Could you check a few things on this model? Use its own coordinates, in mm. Face numbers are marked on the shaded views. A direction names the side the tool comes from. Coordinates: 2 decimals unless noted, no trailing zeros. Loops run counter-clockwise (first coordinate to the right, second up) from the corner with the lowest first, then second, coordinate; pieces in that order, holes last. Notation, with made-up numbers: (45, 6.5) -> (53, 6.5) arc R19 cw to (53, 38.5) -> close; hole circle Ø11 at (44, -37.5). An arc over 180 degrees is marked (long way). One line per question, with ' | ' between items.
from build123d import *

# Parameters (mm, degrees)
CUT_EXTRUDE1_REACH                  = 16.116
CUT_EXTRUDE1_END_RADIUS             = 2.5
CUT_EXTRUDE1_DIRECTION_2_REACH      = 16.116
CUT_EXTRUDE1_DIRECTION_2_END_RADIUS = 2.5


with BuildPart() as part:
    # Sketch2 → Revolve1 (revolve)
    with BuildSketch(Plane.XY):
        with BuildLine():
            Line((3.217141588, 1.1), (4.774934555, 1.1))
            ThreePointArc((4.774934555, 1.1), (4.9, 0), (4.774934555, -1.1))
            Line((4.774934555, -1.1), (3.217141588, -1.1))
            ThreePointArc((3.217141588, -1.1), (3.4, 0), (3.217141588, 1.1))
        make_face()
    revolve(axis=Axis((0, 4.071851736, 0), (0, -1, 0)))

    # Sketch3 → Revolve2 (revolve)
    with BuildSketch(Plane(origin=(0, 0, 0), x_dir=(1, 0, 0), z_dir=(0, 1, 0))):
        with BuildLine():
            Line((-13, 1.5), (-5.974934555, 1.5))
            Line((-5.974934555, 1.5), (-5.974934555, 0))
            Line((-5.974934555, 0), (-4.774934555, 0))
            ThreePointArc((-4.774934555, 0), (-4.594847185, 1.298991664), (-4.068169121, 2.5))
            Line((-4.068169121, 2.5), (-13, 2.5))
            Line((-13, 2.5), (-13, 1.5))
        make_face()
    revolve(axis=Axis((-1.070003769, 0, 0), (-1, 0, 0)))

    # Cut-Extrude1: up to this cylinder (the profile starts inside it)
    cut_extrude1_end = Plane(origin=(-4.461396, 0, 0), z_dir=(1, 0, 0)) * Cylinder(CUT_EXTRUDE1_END_RADIUS, 38.232024, mode=Mode.PRIVATE)
    # Sketch5 → Cut-Extrude1 (cut, up to the surface)
    with BuildSketch(Plane.XY, mode=Mode.PRIVATE) as cut_extrude1_sk1:
        with BuildLine():
            Line((-5.802324208, 2.5), (-3.740894424, 2.5))
            Line((-3.740894424, 2.5), (-3.740894424, 1.1))
            Line((-3.740894424, 1.1), (-4.646504062, 1.1))
            add(Edge.make_bspline(
                [(-4.646504062, 1.1), (-4.808494897, 1.1), (-5.037328654, 1.452538147), (-5.179468889, 2.019128522), (-5.472528246, 2.5), (-5.802324208, 2.5)],
                knots=[0, 0, 0, 0, 0.209972055, 0.594973977, 1, 1, 1, 1], degree=3))
        make_face()
    cut_extrude1_tool1 = extrude(cut_extrude1_sk1.sketch, amount=-CUT_EXTRUDE1_REACH, mode=Mode.PRIVATE) & cut_extrude1_end
    add(cut_extrude1_tool1.solids().sort_by_distance((-4.461384, 1.858771, 0))[0], mode=Mode.SUBTRACT)
    # Sketch5 → Cut-Extrude1 (cut, up to the surface)
    with BuildSketch(Plane.XY, mode=Mode.PRIVATE) as cut_extrude1_sk2:
        with BuildLine():
            Line((-3.740894424, -1.1), (-4.646504062, -1.1))
            add(Edge.make_bspline(
                [(-4.646504062, -1.1), (-4.808494897, -1.1), (-5.037328654, -1.452538147), (-5.179468889, -2.019128522), (-5.472528246, -2.5), (-5.802324208, -2.5)],
                knots=[0, 0, 0, 0, 0.209972055, 0.594973977, 1, 1, 1, 1], degree=3))
            Line((-5.802324208, -2.5), (-3.740894424, -2.5))
            Line((-3.740894424, -2.5), (-3.740894424, -1.1))
        make_face()
    cut_extrude1_tool2 = extrude(cut_extrude1_sk2.sketch, amount=-CUT_EXTRUDE1_REACH, mode=Mode.PRIVATE) & cut_extrude1_end
    add(cut_extrude1_tool2.solids().sort_by_distance((-4.461408, -1.858734, 0))[0], mode=Mode.SUBTRACT)

    # Cut-Extrude1 direction 2: up to this cylinder (the profile starts inside it)
    cut_extrude1_direction_2_end = Plane(origin=(-4.461396, 0, 0), z_dir=(1, 0, 0)) * Cylinder(CUT_EXTRUDE1_DIRECTION_2_END_RADIUS, 38.232024, mode=Mode.PRIVATE)
    # Sketch5 → Cut-Extrude1 direction 2 (cut, up to the surface)
    with BuildSketch(Plane.XY, mode=Mode.PRIVATE) as cut_extrude1_direction_2_sk1:
        with BuildLine():
            Line((-5.802324208, 2.5), (-3.740894424, 2.5))
            Line((-3.740894424, 2.5), (-3.740894424, 1.1))
            Line((-3.740894424, 1.1), (-4.646504062, 1.1))
            add(Edge.make_bspline(
                [(-4.646504062, 1.1), (-4.808494897, 1.1), (-5.037328654, 1.452538147), (-5.179468889, 2.019128522), (-5.472528246, 2.5), (-5.802324208, 2.5)],
                knots=[0, 0, 0, 0, 0.209972055, 0.594973977, 1, 1, 1, 1], degree=3))
        make_face()
    cut_extrude1_direction_2_tool1 = extrude(cut_extrude1_direction_2_sk1.sketch, amount=CUT_EXTRUDE1_DIRECTION_2_REACH, mode=Mode.PRIVATE) & cut_extrude1_direction_2_end
    add(cut_extrude1_direction_2_tool1.solids().sort_by_distance((-4.461384, 1.858771, 0))[0], mode=Mode.SUBTRACT)
    # Sketch5 → Cut-Extrude1 direction 2 (cut, up to the surface)
    with BuildSketch(Plane.XY, mode=Mode.PRIVATE) as cut_extrude1_direction_2_sk2:
        with BuildLine():
            Line((-3.740894424, -1.1), (-4.646504062, -1.1))
            add(Edge.make_bspline(
                [(-4.646504062, -1.1), (-4.808494897, -1.1), (-5.037328654, -1.452538147), (-5.179468889, -2.019128522), (-5.472528246, -2.5), (-5.802324208, -2.5)],
                knots=[0, 0, 0, 0, 0.209972055, 0.594973977, 1, 1, 1, 1], degree=3))
            Line((-5.802324208, -2.5), (-3.740894424, -2.5))
            Line((-3.740894424, -2.5), (-3.740894424, -1.1))
        make_face()
    cut_extrude1_direction_2_tool2 = extrude(cut_extrude1_direction_2_sk2.sketch, amount=CUT_EXTRUDE1_DIRECTION_2_REACH, mode=Mode.PRIVATE) & cut_extrude1_direction_2_end
    add(cut_extrude1_direction_2_tool2.solids().sort_by_distance((-4.461408, -1.858734, 0))[0], mode=Mode.SUBTRACT)


solid = part.part
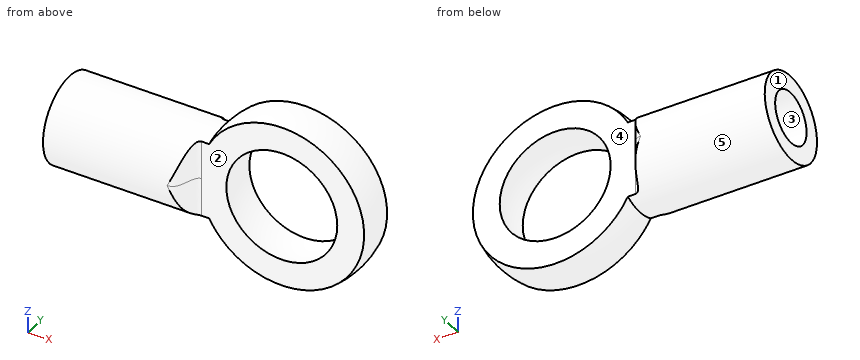
1) I'm going to push flat-ended pins straight in: pin 1 Ø4.5 at (x, z) = (0, -1.5) entering from -Y; pin 2 Ø2 at (x, z) = (-4.5, 1.5) entering from -Y; pin 3 Ø3 at (x, y) = (2.5, -2) entering from -Z. Where does each tip first touch, or does it pass through?
Data:
pin 1: y = -1.1 | pin 2: y = -2.29 | pin 3: z = -4.6
2) If we section it at A-A on y = 0: Please give me the cut outline in (x, z), and give its area (3 significant figures).
Data:
outline: (-13, -2.5) -> (-4.21, -2.5) arc R4.9 ccw (long way) to (-4.21, 2.5) -> (-13, 2.5) -> (-13, 1.5) -> (-5.97, 1.5) -> (-5.97, -1.5) -> (-13, -1.5) -> close; hole circle Ø6.8 at (0, 0) | area: 59.6 mm²
3) If we section it at B-B on z = 3: Please give me the cut outline in (x, y), and give its area (3 significant figures).
Data:
outline: (-3.71, -1.1) -> (-1.16, -1.1) arc R1.6 cw to (-1.16, 1.1) -> (-3.71, 1.1) arc R3.87 ccw to start; (1.16, -1.1) -> (3.71, -1.1) arc R3.87 ccw to (3.71, 1.1) -> (1.16, 1.1) arc R1.6 cw to start | area: 10.4 mm²
4) If we section it at D-D on y = -0.8: Please give me the cut outline in (x, z), and give its area (3 significant figures).
Data:
outline: (-13, -2.37) -> (-4.21, -2.37) arc R4.83 ccw (long way) to (-4.21, 2.37) -> (-13, 2.37) -> (-13, 1.27) -> (-5.97, 1.27) -> (-5.97, -1.27) -> (-13, -1.27) -> close; hole circle Ø6.61 at (0, 0) | area: 60.9 mm²
5) If we section it at C-C on x = 0.25: Please give me the cut outline in (y, z).
Data:
outline: (-1.1, -4.77) arc R4.89 ccw to (1.1, -4.77) -> (1.1, -3.21) arc R3.39 cw to (-1.1, -3.21) -> close; (-1.1, 3.21) arc R3.39 cw to (1.1, 3.21) -> (1.1, 4.77) arc R4.89 ccw to (-1.1, 4.77) -> close
6) On a 3-axis mill with a long thin cutter (end or side, diameter ignored), from which of +Z, -Z, +X, -X, +Y, -Y can I reach the whole of each face in a straight line? I mean the marked faces 1 and 2. Say none if no direction works.
Data:
face 1: +Z, -Z, -X, +Y, -Y | face 2: +Z, -Z, +X, -Y
7) We'd pull the mould along Z, two halves only. Please class the marked faces 3, 4 and 5: pulls with the +Z half, pulls with the -Z half, needs draft (parallel to the pull), parting line crosses it, or undercut.
Data:
face 3: undercut | face 4: needs draft | face 5: parting line crosses it
8) I need wall thicknesses on line 1 along Z through (x, y) = (-8.5, 0); line 2 along Z through (x, y) = (-11, -0.75). Which ranges of each line are inside material? Lowest first, please. Write a range as from..to.
Data:
line 1: -2.5..-1.5, 1.5..2.5 | line 2: -2.38..-1.3, 1.3..2.38
